The figure shows three views and two pictorial views of one solid part (mm, origin at its lowest corner). Answer the questions. Give positions to 0.01 mm unless a question says otherwise; leave off trailing zeros. Order: outer loops, then holes, each group sorted by start corner. A loop starts at its lowest first (then second) coordinate and runs counter-clockwise, first axis right, second up. Notation, with made-up numbers: M 32.25,61 L 38.25,61 A22 ccw 38.25,69 Z; hole C 46.5,-12.5 d4. An arc over 180 degrees is marked long. One line per item, written item: value.
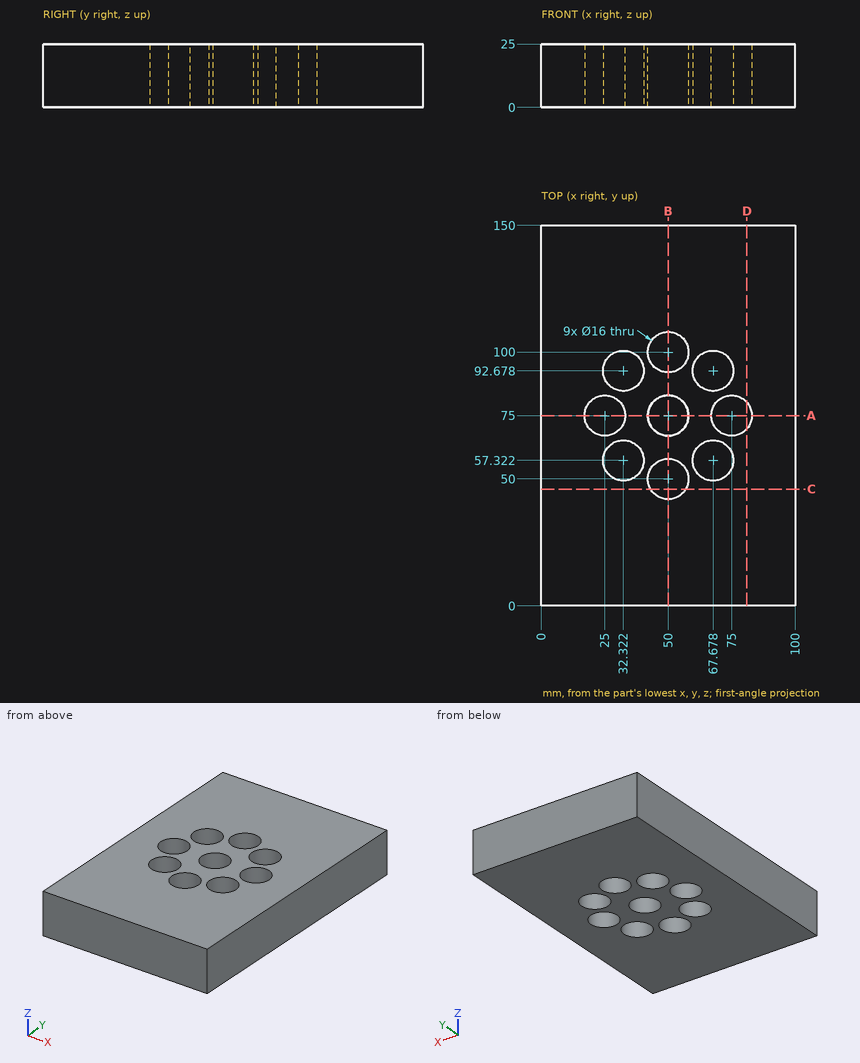
1) Each of these flat-tipped pins is pushed along its axis until it touches: pin 1 Ø21 at (x, y) = (50, 75) entering from -Z; pin 2 Ø9.5 at (x, y) = (32.32, 57.32) entering from -Z. Where does it stop, or does it pass through?
Reported:
pin 1: stops at z = 0
pin 2: passes through
2) Find section A-A, the plane y = 75. Write down the section's boundary in (x, z).
Reported:
outline: M 0,0 L 17,0 L 17,25 L 0,25 Z; M 33,0 L 42,0 L 42,25 L 33,25 Z; M 58,0 L 67,0 L 67,25 L 58,25 Z; M 83,0 L 100,0 L 100,25 L 83,25 Z
3) Find section C-C, the plane y = 46. Write down the section's boundary in (x, z), plus the area to 3 significant figures.
Reported:
outline: M 0,0 L 43.07,0 L 43.07,25 L 0,25 Z; M 56.93,0 L 100,0 L 100,25 L 56.93,25 Z
area: 2,150 mm^2
4) Consider probe 1 along Y at (x, z) = (52, 12.5) (1 decimal); probe 2 along Y at (x, z) = (30, 20) (1 decimal); probe 3 along X at (y, z) = (50, 15.5) (1 decimal). Determine where each line is inside the solid, lowest interval first.
Reported:
probe 1: y = 0 to 42.3, 57.7 to 67.3, 82.7 to 92.3, 107.7 to 150
probe 2: y = 0 to 49.7, 65 to 68.8, 81.2 to 85, 100.3 to 150
probe 3: x = 0 to 29.1, 35.5 to 42, 58 to 64.5, 70.9 to 100
5) Find section D-D, the plane x = 81. Write down the section's boundary in (y, z).
Reported:
outline: M 0,0 L 69.71,0 L 69.71,25 L 0,25 Z; M 80.29,0 L 150,0 L 150,25 L 80.29,25 Z
6) Find section B-B, the plane x = 50. Write down the section's boundary in (y, z).
Reported:
outline: M 0,0 L 42,0 L 42,25 L 0,25 Z; M 58,0 L 67,0 L 67,25 L 58,25 Z; M 83,0 L 92,0 L 92,25 L 83,25 Z; M 108,0 L 150,0 L 150,25 L 108,25 Z
